Autodesk Inventor part; units mm, degrees
ref_plane "YZ Plane" through (0, 0, 0) normal (1, 0, 0) x (0, 1, 0)
ref_plane "XZ Plane" through (0, 0, 0) normal (0, 1, 0) x (-1, 0, 0)
ref_plane "XY Plane" through (0, 0, 0) normal (0, 0, 1) x (1, 0, 0)
sketch "スケッチ1" plane through (0, 0, 0) normal (0, 0, 1) x (1, 0, 0)
  line L0 (-120, 55) -> (120, 55)
  line L1 (120, 55) -> (120, -55)
  line L2 (120, -55) -> (-120, -55)
  line L3 (-120, -55) -> (-120, 55)
  point P0 (0, 0)
  point P1 (0, -55)
  point P2 (120, 0)
  dimension "d0" = 240
  dimension "d1" = 110
extrude "天板" add sketch "スケッチ1" along normal blind 15
sketch "スケッチ2" plane through (0, 0, 15) normal (0, 0, 1) x (1, 0, 0)
  line L0 (-118, 53) -> (118, 53)
  line L1 (118, 53) -> (118, -53)
  line L2 (118, -53) -> (-118, -53)
  line L3 (-118, -53) -> (-118, 53)
  point P0 (0, 0)
  point P1 (0, -53)
  point P2 (118, 0)
  dimension "d4" = 236
  dimension "d5" = 106
extrude "天板くりぬき" cut sketch "スケッチ2" against normal blind 13
sketch "スケッチ3" plane through (0, 0, 2) normal (0, 0, 1) x (1, 0, 0)
  line L0 (-118, 53) -> (-110, 53)
  line L1 (-110, 53) -> (-110, 45)
  line L2 (-110, 45) -> (-118, 45)
  line L3 (-118, 45) -> (-118, 53)
  line L4 (-118, -45) -> (-110, -45)
  line L5 (-110, -45) -> (-110, -53)
  line L6 (-110, -53) -> (-118, -53)
  line L7 (-118, -53) -> (-118, -45)
  line L8 (110, 53) -> (118, 53)
  line L9 (118, 53) -> (118, 45)
  line L10 (118, 45) -> (110, 45)
  line L11 (110, 45) -> (110, 53)
  line L12 (110, -45) -> (118, -45)
  line L13 (118, -45) -> (118, -53)
  line L14 (118, -53) -> (110, -53)
  line L15 (110, -53) -> (110, -45)
  line L16 (-5, 53) -> (5, 53)
  line L17 (5, 53) -> (5, 45)
  line L18 (5, 45) -> (-5, 45)
  line L19 (-5, 45) -> (-5, 53)
  line L20 (-5, -45) -> (5, -45)
  line L21 (5, -45) -> (5, -53)
  line L22 (5, -53) -> (-5, -53)
  line L23 (-5, -53) -> (-5, -45)
  line L24 (-118, 53) -> (118, 53)
  line L25 (118, -53) -> (-118, -53)
  point P0 (0, 0)
  point P1 (0, 53)
  point P2 (0, 53)
  point P3 (0, -53)
  point P4 (0, -53)
  dimension "d8" = 8
  dimension "d9" = 8
  dimension "d10" = 10
extrude "天板固定用ボス" add sketch "スケッチ3" along normal blind 13
sketch "スケッチ4" plane through (0, 0, 15) normal (0, 0, 1) x (1, 0, 0)
  circle A0 centre (-115, 50) radius 1.4
  circle A1 centre (-115, -50) radius 1.4
  circle A2 centre (0, -50) radius 1.4
  circle A3 centre (0, 50) radius 1.4
  circle A4 centre (115, 50) radius 1.4
  circle A5 centre (115, -50) radius 1.4
  line L0 (120, 55) -> (-120, 55)
  line L1 (-120, 55) -> (-120, -55)
  line L2 (-120, -55) -> (120, -55)
  line L3 (120, 55) -> (120, -55)
  point P0 (0, 0)
  dimension "d13" = 2.8
  dimension "d14" = 5
  dimension "d15" = 5
  dimension "d16" = 5
  dimension "d17" = 5
extrude "天板固定用ねじ穴" cut sketch "スケッチ4" against normal blind 10 contours A0 | A1 | A2 | A3 | A4 | A5
sketch "スケッチ5" plane through (0, 0, 2) normal (0, 0, 1) x (1, 0, 0)
  line L0 (-34.5, 35.5) -> (110.5, 35.5)
  line L1 (110.5, 35.5) -> (110.5, -35.5)
  line L2 (110.5, -35.5) -> (-34.5, -35.5)
  line L3 (-34.5, -35.5) -> (-34.5, 35.5)
  line L4 (-85, 34.5) -> (-111, 34.5)
  line L5 (-111, 34.5) -> (-111, 23.5)
  line L6 (-111, 23.5) -> (-85, 23.5)
  line L7 (-85, 23.5) -> (-85, 34.5)
  point P0 (0, 0)
  point P1 (-10, 0)
  point P2 (86, 0)
  point P3 (38, 0)
  point P4 (38, 35.5)
  point P5 (-34.5, 0)
  point P6 (-85, 29)
  point P7 (-85, 29)
  dimension "d20" = 10
  dimension "d21" = 96
  dimension "d22" = 145
  dimension "d23" = 71
  dimension "d24" = 48
  dimension "d27" = 85
  dimension "d28" = 29
  dimension "d31" = 26
  dimension "d32" = 11
extrude "7セグ LCD用穴" cut sketch "スケッチ5" against normal blind 2
fillet "フィレット1" radius 3 4 edges at (120, -55, 7.5) (120, 55, 7.5) (-120, -55, 7.5) (-120, 55, 7.5)
sketch "スケッチ6" plane through (0, 0, 2) normal (0, 0, 1) x (1, 0, 0)
  line L0 (-114, 37.5) -> (-74, 37.5)
  line L1 (-74, 37.5) -> (-74, 12.5)
  line L2 (-74, 12.5) -> (-114, 12.5)
  line L3 (-114, 12.5) -> (-114, 37.5)
  line L4 (-85, 34.5) -> (-85, 23.5)
  line L5 (-111, 23.5) -> (-111, 34.5)
  point P0 (0, 0)
  point P1 (-74, 25)
  point P2 (-85, 29)
  dimension "d34" = 40
  dimension "d35" = 25
  dimension "d36" = 3
  dimension "d55" = 4
extrude "LCD用くぼみ" cut sketch "スケッチ6" against normal blind 1.2
sketch "スケッチ8" plane through (-120, -52, 0) normal (-1, 0, 0) x (0, 0, 1)
  line L0 (0, 16.5) -> (0, 87.5)
  line L1 (15, 0) -> (15, 104)
  line L2 (15, 61.38) -> (13, 61.38)
  line L3 (13, 61.38) -> (13, 50.38)
  line L4 (13, 50.38) -> (15, 50.38)
  line L5 (15, 50.38) -> (15, 61.38)
  line L6 (15, 31.9) -> (13, 31.9)
  line L7 (13, 31.9) -> (13, 18.9)
  line L8 (13, 18.9) -> (15, 18.9)
  line L9 (15, 18.9) -> (15, 31.9)
  point P0 (0, 52)
  point P1 (0, 63.5)
  point P2 (15, 55.88)
  point P3 (15, 25.4)
  point P4 (15, 55.88)
  point P5 (15, 25.4)
  dimension "d46" = 11.5
  dimension "d47" = 7.62
  dimension "d48" = 38.1
  dimension "d49" = 2
  dimension "d50" = 11
  dimension "d51" = 2
  dimension "d52" = 13
extrude "Arduinoコネクタ穴" cut sketch "スケッチ8" against normal blind 2
properties part number "top-cover"
Geometry check sheet. Reference: the model listing, model coordinates, mm. Give positions to 0.01 mm unless a question says otherwise; leave off trailing zeros. Loops run counter-clockwise (first coordinate to the right, second up) from the corner with the lowest first, then second, coordinate; pieces in that order, holes last. Notation, with made-up numbers: M 29,22.5 L 48,22.5 A27 ccw 48,53.5 Z; hole C 61,-13.5 d9. An arc over 180 degrees is marked long. Write item = value, one per line. Start each with the question number.
1. Section check D-D, the plane x = -82.5. Enter the section's corners in (y, z).
2. Draft check along X on faces 1 (the face through (-58, 53, 9)), 2 (the face through (-120, -1, 7)), 3 (the face through (-9.4, 53.2, 15)). Enter one of: +X half, -X half, draft (parallel to the pull), parting line (faces both ways), or undercut.
3. Go/stop test with flat-tipped pins: P1, Ø3, axis at x = -115.5, y = 49.5, coming from the +Z side; P2, Ø1, axis at x = -35.5, y = 5.5, coming from the +Z side; P3, Ø1.6, axis at x = -118.5, y = 6.5, coming from the +Z side. Record where each tip stops, or that it passes through.
4. Section check C-C, the plane y = 26. Enter the section's corners in (x, z), plus the area to 3 significant figures.
5. Thickness scan on probe 1 along X at (y, z) = (47, 5.75); probe 2 along Y at (x, z) = (-115, 10); probe 3 along X at (y, z) = (2.5, 2.25). Record the ranges inside material, lowest first.
6. Section check A-A, the plane x = 69. Enter the section's corners in (y, z), plus the area to 3 significant figures.
7. Section check B-B, the plane y = 6. Enter the section's corners in (x, z), plus the area to 3 significant figures.
Values follow:
q1.outline = M -55,0 L 55,0 L 55,15 L 53,15 L 53,2 L 37.5,2 L 37.5,0.8 L 12.5,0.8 L 12.5,2 L -53,2 L -53,15 L -55,15 Z
q2.face_1 = undercut
q2.face_2 = -X half
q2.face_3 = draft
q3.P1 = 15
q3.P2 = 2
q3.P3 = 13
q4.outline = M -120,0 L -111,0 L -111,0.8 L -114,0.8 L -114,2 L -118,2 L -118,15 L -120,15 Z; M -85,0 L -34.5,0 L -34.5,2 L -74,2 L -74,0.8 L -85,0.8 Z; M 110.5,0 L 120,0 L 120,15 L 118,15 L 118,2 L 110.5,2 Z
q4.area = 173 mm^2
q5.probe_1 = -120 to -110, -5 to 5, 110 to 120
q5.probe_2 = -55 to -51.4, -48.6 to -45, 45 to 48.6, 51.4 to 55
q5.probe_3 = -120 to -118, 118 to 120
q6.outline = M -55,0 L -35.5,0 L -35.5,2 L -53,2 L -53,15 L -55,15 Z; M 35.5,0 L 55,0 L 55,15 L 53,15 L 53,2 L 35.5,2 Z
q6.area = 130 mm^2
q7.outline = M -120,0 L -34.5,0 L -34.5,2 L -118,2 L -118,13 L -120,13 Z; M 110.5,0 L 120,0 L 120,15 L 118,15 L 118,2 L 110.5,2 Z
q7.area = 238 mm^2
